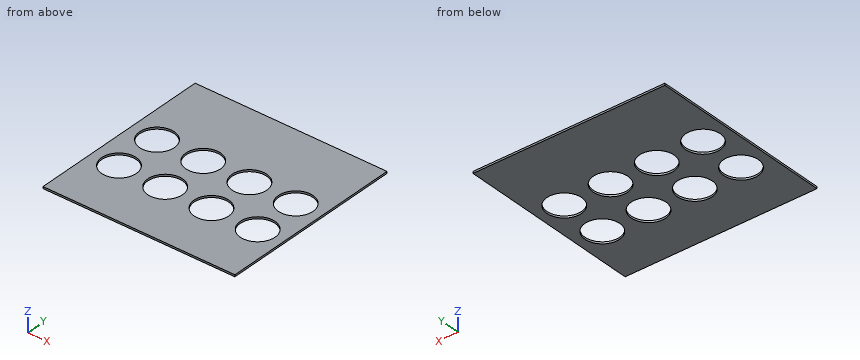
Autodesk Inventor part; units mm, degrees
ref_plane "YZ Plane" through (0, 0, 0) normal (1, 0, 0) x (0, 1, 0)
ref_plane "XZ Plane" through (0, 0, 0) normal (0, 1, 0) x (-1, 0, 0)
ref_plane "XY Plane" through (0, 0, 0) normal (0, 0, 1) x (1, 0, 0)
sketch "Sketch1" plane through (0, 0, 0) normal (0, 0, 1) x (1, 0, 0)
  line L0 (-41.9595, 102.9157) -> (590.5005, 102.9157)
  line L1 (590.5005, 102.9157) -> (590.5005, 712.5157)
  line L2 (590.5005, 712.5157) -> (-41.9595, 712.5157)
  line L3 (-41.9595, 712.5157) -> (-41.9595, 102.9157)
  line L4 (-41.9595, 712.5157) -> (-23.3159, 712.5157)
  line L5 (590.5005, 712.5157) -> (546.0505, 712.5157)
  line L6 (546.0505, 712.5157) -> (406.3505, 712.5157)
  line L7 (406.3505, 712.5157) -> (393.6505, 712.5157)
  line L8 (393.6505, 712.5157) -> (253.9505, 712.5157)
  line L9 (253.9505, 712.5157) -> (241.2505, 712.5157)
  line L10 (241.2505, 712.5157) -> (101.5505, 712.5157)
  line L11 (101.5505, 712.5157) -> (88.8505, 712.5157)
  line L12 (88.8505, 712.5157) -> (-23.3159, 712.5157)
  line L13 (590.5005, 102.9157) -> (590.5005, 229.9157)
  line L14 (590.5005, 229.9157) -> (590.5005, 369.6157)
  line L15 (590.5005, 369.6157) -> (590.5005, 382.3157)
  line L16 (590.5005, 382.3157) -> (590.5005, 522.0157)
  circle A0 centre (46.5341, 452.1657) radius 57.15
  circle A1 centre (198.9341, 452.1657) radius 57.15
  circle A2 centre (351.3341, 452.1657) radius 57.15
  circle A3 centre (503.7341, 452.1657) radius 57.15
  circle A4 centre (46.5341, 299.7657) radius 57.15
  circle A5 centre (198.9341, 299.7657) radius 57.15
  circle A6 centre (351.3341, 299.7657) radius 57.15
  circle A7 centre (503.7341, 299.7657) radius 57.15
  line L17 (-23.3159, 712.5157) -> (116.3841, 712.5157)
  line L18 (116.3841, 712.5157) -> (129.0841, 712.5157)
  line L19 (129.0841, 712.5157) -> (268.7841, 712.5157)
  line L20 (268.7841, 712.5157) -> (281.4841, 712.5157)
  line L21 (281.4841, 712.5157) -> (421.1841, 712.5157)
  line L22 (421.1841, 712.5157) -> (433.8841, 712.5157)
  line L23 (433.8841, 712.5157) -> (573.5841, 712.5157)
  dimension "d0" = 632.46
  dimension "d1" = 609.6
  dimension "d2" = 18.6436
  dimension "d24" = 127
  dimension "d25" = 139.7
  dimension "d26" = 12.7
  dimension "d27" = 139.7
  dimension "d28" = 114.3
  dimension "d29" = 114.3
  dimension "d30" = 114.3
  dimension "d31" = 114.3
  dimension "d32" = 114.3
  dimension "d33" = 114.3
  dimension "d34" = 114.3
  dimension "d35" = 114.3
  dimension "d38" = 139.7
  dimension "d39" = 12.7
  dimension "d40" = 139.7
  dimension "d41" = 12.7
  dimension "d42" = 139.7
  dimension "d43" = 12.7
  dimension "d44" = 139.7
extrude "Extrusion2" add sketch "Sketch1" along normal blind 6.35
equation "\"BendRadius\" = Thickness"
equation "\"BendReliefWidth\" = Thickness"
equation "\"BendReliefDepth\" = 0.5 * Thickness"
equation "\"CornerReliefSize\" = 4 * Thickness"
equation "\"MinimumRemnant\" = 2 * Thickness"
equation "\"TransitionRadius\" = BendRadius"
equation "\"JacobiRadiusSize\" = BendRadius"
equation "\"GapSize\" = Thickness"
properties part number "vessel support top"
The model under review builds one solid part; all positions refer to its coordinate system, in mm. Round coordinates to 2 decimals unless told otherwise and drop trailing zeros. Loops run counter-clockwise (first coordinate to the right, second up) from the corner with the lowest first, then second, coordinate; pieces in that order, holes last. Notation, with made-up numbers: M 82,17 L 125,17 A22 cw 125,24 Z; hole C 61,-0.5 d6. An arc over 180 degrees is marked long. Write item = value, one per line.
Item 1: Take a section at B-B on z = 4.25. State how many separate pieces and enclosed holes the cut face has, then the cut area to 3 significant figures.
Return value:
separate_pieces = 1
enclosed_holes = 8
area = 303,000 mm2
Item 2: Take a section at C-C on x = 219. Write out the cut boundary in (y, z), then the cut area to 3 significant figures.
Return value:
outline = M 102.92,0 L 246.25,0 L 246.25,6.35 L 102.92,6.35 Z; M 353.28,0 L 398.65,0 L 398.65,6.35 L 353.28,6.35 Z; M 505.68,0 L 712.52,0 L 712.52,6.35 L 505.68,6.35 Z
area = 2,510 mm2
Item 3: Take a section at A-A on x = 473. Write out the cut boundary in (y, z).
Return value:
outline = M 102.92,0 L 251.58,0 L 251.58,6.35 L 102.92,6.35 Z; M 347.95,0 L 403.98,0 L 403.98,6.35 L 347.95,6.35 Z; M 500.35,0 L 712.52,0 L 712.52,6.35 L 500.35,6.35 Z
Item 4: For line 1 (Y direction, x = 459, z = 2.25); line 2 (Y direction, x = 25, z = 2.25); line 3 (X direction, y = 352, z = 2.25), list the stretches that pass through material, from the lowest coordinate up. Write a range as [from, to].
Return value:
line_1 = [102.92, 264.2], [335.33, 416.6], [487.73, 712.52]
line_2 = [102.92, 246.83], [352.7, 399.23], [505.1, 712.52]
line_3 = [-41.96, 23.35], [69.72, 175.75], [222.12, 328.15], [374.52, 480.55], [526.92, 590.5]
